Could you check a few things on this drawing? It's one solid part, dimensions in mm from its lowest x, y, z. A direction names the side the tool comes from. Coordinates: 2 decimals unless noted, no trailing zeros. Loops run counter-clockwise (first coordinate to the right, second up) from the corner with the lowest first, then second, coordinate; pieces in that order, holes last. Notation, with made-up numbers: M 78.25,25 L 137.25,25 A7 ccw 137.25,33 Z; hole C -12,-37 d9. An arc over 180 degrees is marked long. Use one line per item in the form item = value. Start each with the question number.
(1) Imagine slicing it at C-C, the plane x = 1.5. Please give me the cut outline in (y, z).
(2) Please list where these lines run through material, in increasing order: L1, parallel to X at y = 13, z = 20.75; L2, parallel to Z at x = 0.5, y = 15; L3, parallel to Y at x = 9.5, z = 12.25.
(3) Will these pins go through, and if not, where does the flat tip stop? P1, Ø8, axis at y = 5.5, z = 16, coming from the -X side; P2, Ø6, axis at x = 1.5, y = 5.5, coming from the -Z side; P3, Ø1.6, axis at x = 1, y = 14.5, coming from the -Z side; P4, Ø1.6, axis at x = 0.5, z = 20, coming from the -Y side.
(4) Imagine slicing it at A-A, the plane y = 13.25. Please give me the cut outline in (x, z), and give its area (3 significant figures).
(5) On a 3-axis mill with a long thin cutter (end or side, diameter ignored), from which of +Z, -Z, +X, -X, +Y, -Y can I reach the whole of each face in a straight line? I mean the marked faces 4 and 5. Say none if no direction works.
(6) Imagine slicing it at D-D, the plane y = 1.75. Please give me the cut outline in (x, z), and give its area (3 significant figures).
(7) Imagine slicing it at B-B, the plane z = 19.25. Please give me the cut outline in (x, y), and give its area (4 significant figures).
(8) Thinking about a two-plate mould opening in X: for the marked faces 1, 2 and 3, which applies, +X half, -X half, draft (parallel to the pull), parting line (faces both ways), or undercut?
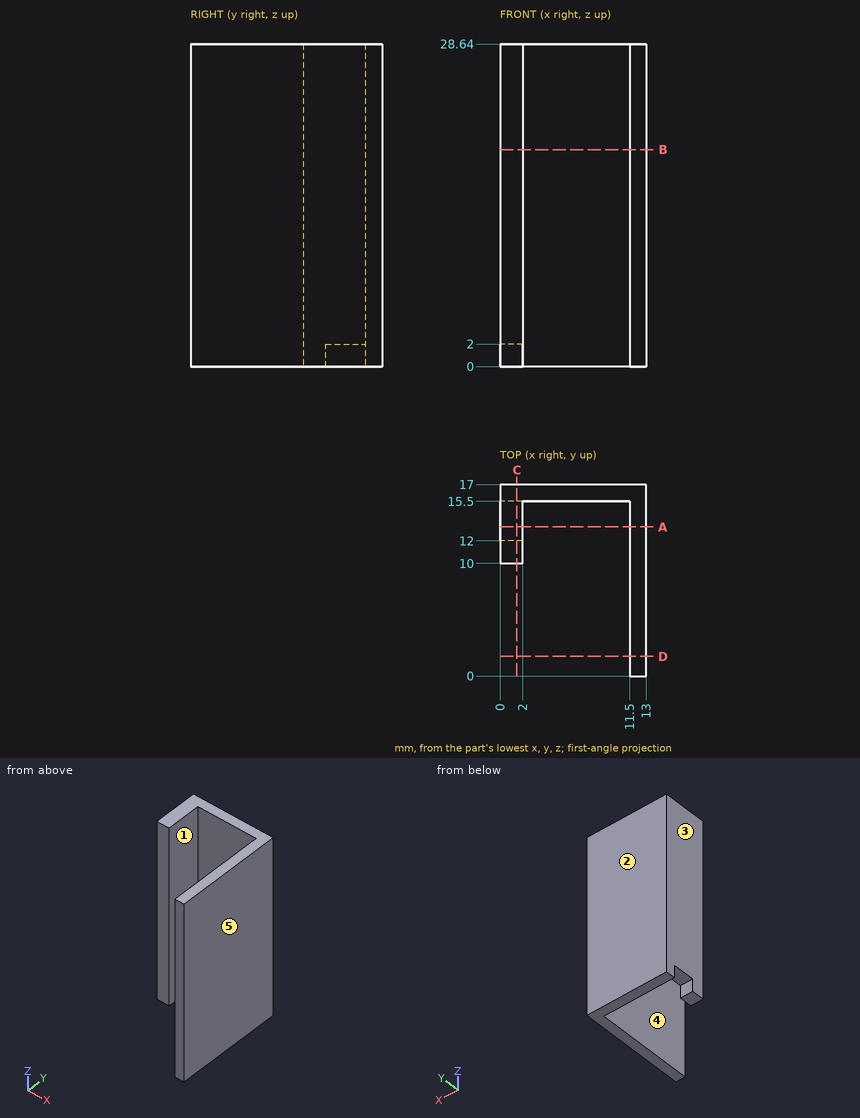
Answer:
q1.outline = M 10,0 L 12,0 L 12,2 L 15.5,2 L 15.5,0 L 17,0 L 17,28.64 L 10,28.64 Z
q2.L1 = 0 to 2, 11.5 to 13
q2.L2 = 2 to 28.64
q2.L3 = 15.5 to 17
q3.P1 = 11.5
q3.P2 = through
q3.P3 = 2
q3.P4 = 10
q4.outline = M 0,2 L 2,2 L 2,28.64 L 0,28.64 Z; M 11.5,0 L 13,0 L 13,28.64 L 11.5,28.64 Z
q4.area = 96.2 mm²
q5.face_4 = +Z, -Z, -Y
q5.face_5 = +Z, -Z, +X, +Y, -Y
q6.outline = M 11.5,0 L 13,0 L 13,28.64 L 11.5,28.64 Z
q6.area = 43.0 mm²
q7.outline = M 0,10 L 2,10 L 2,15.5 L 11.5,15.5 L 11.5,0 L 13,0 L 13,17 L 0,17 Z
q7.area = 53.75 mm²
q8.face_1 = undercut
q8.face_2 = draft
q8.face_3 = -X half
